```python
from build123d import *

# Parameters (mm, degrees)
SKETCH1_W             = 85
SKETCH1_H             = 85
BOSS_EXTRUDE1_DEPTH   = 3.175
SKETCH2_R             = 1.985
CUT_EXTRUDE1_DEPTH    = 121.250075364
LPATTERN1_COUNT       = 2
LPATTERN1_PITCH       = 65.09
LPATTERN1_COUNT_DIR2  = 2
LPATTERN1_PITCH_DIR2  = 65.09
FILLET1_R             = 3.175
SKETCH3_R             = 3.5
CUT_EXTRUDE2_DEPTH    = 121.250075364
M3X0_5_TAPPED_HOLE1_D = 2.5


with BuildPart() as part:
    # Sketch1 → Boss-Extrude1 (new body)
    with BuildSketch(Plane(origin=(0, 0, 0), x_dir=(1, 0, 0), z_dir=(0, 1, 0))):
        with Locations((42.5, 42.5)):
            Rectangle(SKETCH1_W, SKETCH1_H)
    extrude(amount=BOSS_EXTRUDE1_DEPTH)

    # Sketch2 → Cut-Extrude1 (cut, through all)
    with BuildSketch(Plane(origin=(0, 3.175, 0), x_dir=(1, 0, 0), z_dir=(0, 1, 0))):
        with Locations(Location((9.955, 75.045, 0), (0, 0, 270))):
            Circle(SKETCH2_R)
    cut_extrude1 = extrude(amount=-CUT_EXTRUDE1_DEPTH, mode=Mode.SUBTRACT)

    # LPattern1: Cut-Extrude1 2 × 2
    with Locations(*[(j * LPATTERN1_PITCH_DIR2, 0, i * LPATTERN1_PITCH) for i in range(LPATTERN1_COUNT) for j in range(LPATTERN1_COUNT_DIR2) if (i, j) != (0, 0)]):
        add(cut_extrude1, mode=Mode.SUBTRACT)

    # Fillet1
    fillet1_edges = [part.edges().sort_by_distance(p)[0] for p in [
        (0, 1.5875, -85),
        (85, 1.5875, -85),
        (85, 1.5875, 0),
        (0, 1.5875, 0),
    ]]
    fillet(fillet1_edges, radius=FILLET1_R)

    # Sketch3 → Cut-Extrude2 (cut, through all)
    with BuildSketch(Plane(origin=(0, 3.175, 0), x_dir=(1, 0, 0), z_dir=(0, 1, 0))):
        with Locations(Location((42.5, 42.5, 0), (0, 0, 270))):
            Circle(SKETCH3_R)
    extrude(amount=-CUT_EXTRUDE2_DEPTH, mode=Mode.SUBTRACT)

    # M3x0.5 Tapped Hole1 (through all)
    with Locations(Plane(origin=(0, 3.175, 0), x_dir=(1, 0, 0), z_dir=(0, 1, 0))):
        with Locations((34, 42.5), (51, 42.5)):
            Hole(M3X0_5_TAPPED_HOLE1_D / 2)


solid = part.part
```
Verification items for the finished model (mm, model axes). Give positions to 0.01 mm unless a question says otherwise; leave off trailing zeros. Order: outer loops, then holes, each group sorted by start corner. A loop starts at its lowest first (then second) coordinate and runs counter-clockwise, first axis right, second up. Notation, with made-up numbers: M 35.25,44 L 57.25,44 A16 cw 57.25,59 Z; hole C 66.5,62.5 d11. An arc over 180 degrees is marked long. Answer in a Markdown table with one row per item. Add a question column.
Item 1: Scan lines: probe 1 along X at (y, z) = (0.75, -42.5); probe 2 along Z at (x, y) = (51, 1.2); probe 3 along X at (y, z) = (2.05, -76.5). Record each from-to range of solid material in increasing order. Write a range as from..to.
Item 2: Mould release check, pull along Z, two halves, no side actions. Record for faces 1 (the cylindrical face through (0.91, 1.61, -84.05)), 2 (the flat face through (0, 2, -42)), 3 (the cylindrical face through (9.195, 1.61, -8.121)): released by +Z, released by -Z, zero draft, split by the parting line, or undercut.
Item 3: Section check A-A, the plane x = 34. Enter the section's corners in (y, z) (3 decimals).
Item 4: Section check B-B, the plane z = -42.5. Enter the section's corners in (x, y) (3 decimals), and give its area (3 significant figures).
Filled sheet:
| question | item | result |
|---|---|---|
| 1 | probe 1 | x = 0..32.75, 35.25..39, 46..49.75, 52.25..85 |
| 1 | probe 2 | z = -85..-43.75, -41.25..0 |
| 1 | probe 3 | x = 0..8.6, 11.31..73.69, 76.4..85 |
| 2 | face 1 | released by -Z |
| 2 | face 2 | zero draft |
| 2 | face 3 | undercut |
| 3 | outline | M 0,-85 L 3.175,-85 L 3.175,-43.75 L 0,-43.75 Z; M 0,-41.25 L 3.175,-41.25 L 3.175,0 L 0,0 Z |
| 4 | outline | M 0,0 L 32.75,0 L 32.75,3.175 L 0,3.175 Z; M 35.25,0 L 39,0 L 39,3.175 L 35.25,3.175 Z; M 46,0 L 49.75,0 L 49.75,3.175 L 46,3.175 Z; M 52.25,0 L 85,0 L 85,3.175 L 52.25,3.175 Z |
| 4 | area | 232 mm^2 |
